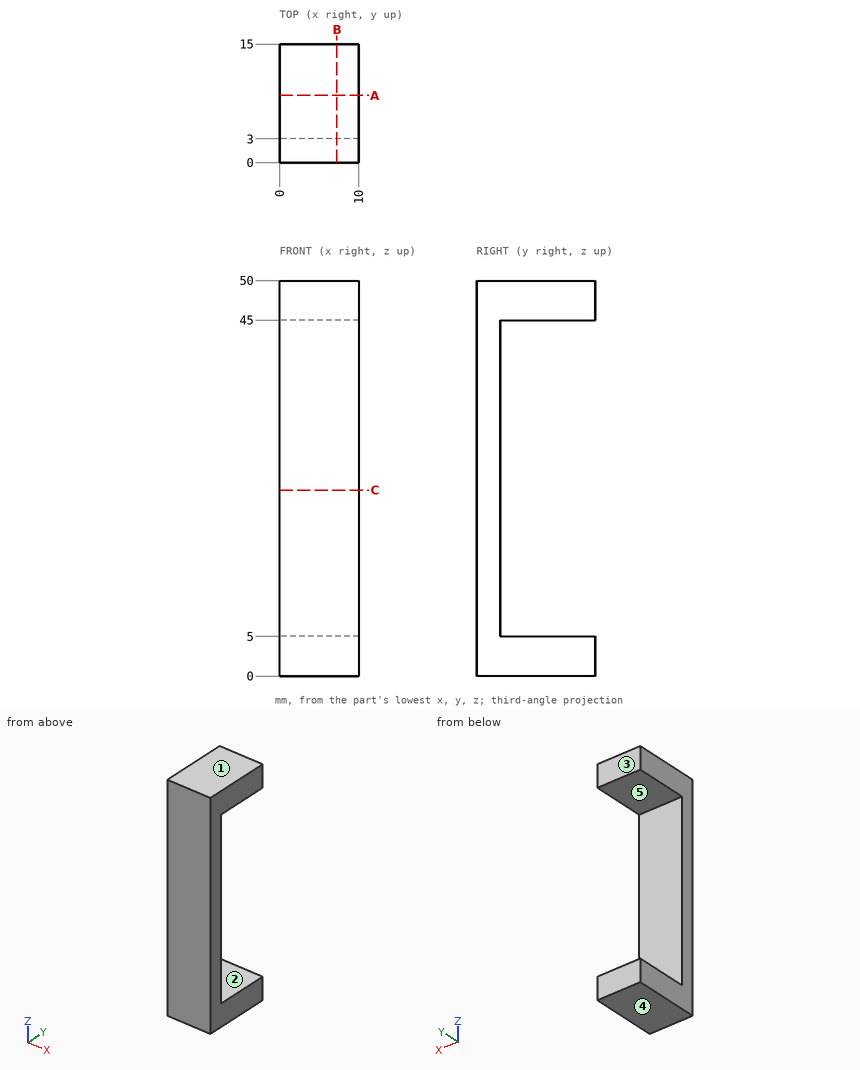
Print and shaded views of the part. All mm, measured from the part's lowest x, y and z. A direction names the side the tool comes from. Give positions to 0.01 mm unless a question says otherwise; leave off trailing zeros. Loops run counter-clockwise (first coordinate to the right, second up) from the corner with the lowest first, then second, coordinate; pieces in that order, holes last. Notation, with made-up numbers: (-31, -20.75) -> (-24, -20.75) arc R18 ccw to (-24, 4.25) -> close; hole circle Ø9 at (21.25, -15.75). An arc over 180 degrees is marked (long way). Use CSV: the item, a comma, the result in double quotes. Start each with the question number.
1) Flat gauge pins, fed straight in: pin 1 Ø5 at (x, z) = (4.5, 19.5) entering from +Y; pin 2 Ø6 at (y, z) = (7, 11.5) entering from +X. Where does each tip first touch, or does it go through?
2) Slice it at A-A on y = 8.5. Give the cut face in (x, z), plus the area to 3 significant figures.
3) Mould opens along Z. For the marked faces 3, 4 and 5 say: released by +Z, released by -Z, zero draft, split by the parting line, or undercut.
4) Slice it at B-B on x = 7.25. Give the cut face in (y, z).
5) Slice it at C-C on z = 23.5. Give the cut face in (x, y).
6) Wall check: line 1 (Z direction, x = 1, y = 13.25); line 2 (Y direction, x = 5.5, z = 23.5). Give the ranges that are in metal, low to high.
7) Tool access for the marked faces 1 and 2: list every direction of +Z, -Z, +X, -X, +Y, -Y with a clear straight run to the whole face (end or side of a thin tool).
Computed values:
1,pin 1,"stops at y = 3"
1,pin 2,"passes through"
2,outline,"(0, 0) -> (10, 0) -> (10, 5) -> (0, 5) -> close; (0, 45) -> (10, 45) -> (10, 50) -> (0, 50) -> close"
2,area,"100 mm^2"
3,face 3,"zero draft"
3,face 4,"released by -Z"
3,face 5,"undercut"
4,outline,"(0, 0) -> (15, 0) -> (15, 5) -> (3, 5) -> (3, 45) -> (15, 45) -> (15, 50) -> (0, 50) -> close"
5,outline,"(0, 0) -> (10, 0) -> (10, 3) -> (0, 3) -> close"
6,line 1,"z = 0 to 5, 45 to 50"
6,line 2,"y = 0 to 3"
7,face 1,"+Z, +X, -X, +Y, -Y"
7,face 2,"+X, -X, +Y"
